```python
from build123d import *

# Parameters (mm, degrees)
SKETCH1_W           = 20
SKETCH1_H           = 50
BOSS_EXTRUDE1_DEPTH = 3
SKETCH2_W           = 50
SKETCH2_H           = 45
SKETCH2_R           = 3.5
BOSS_EXTRUDE2_DEPTH = 3


with BuildPart() as part:
    # Sketch1 → Boss-Extrude1 (new body)
    with BuildSketch(Plane(origin=(0, 0, 0), x_dir=(1, 0, 0), z_dir=(0, 1, 0))):
        Rectangle(SKETCH1_W, SKETCH1_H)
    extrude(amount=BOSS_EXTRUDE1_DEPTH)

    # Sketch2 → Boss-Extrude2 (add)
    with BuildSketch(Plane(origin=(10, 0, 0), x_dir=(0, 0, -1), z_dir=(1, 0, 0))):
        with Locations((0, 22.5)):
            Rectangle(SKETCH2_W, SKETCH2_H)
        with Locations((0, 29)):
            Circle(SKETCH2_R, mode=Mode.SUBTRACT)
    extrude(amount=BOSS_EXTRUDE2_DEPTH)


solid = part.part
```
Can you work these out from the model? Positions are in its coordinate system, mm. A direction names the side the tool comes from. Round coordinates to 2 decimals unless told otherwise and drop trailing zeros. Loops run counter-clockwise (first coordinate to the right, second up) from the corner with the lowest first, then second, coordinate; pieces in that order, holes last.
Item 1: Will these pins go through, and if not, where does the flat tip stop? pin 1 Ø1.5 at (y, z) = (34.5, 7) entering from -X; pin 2 Ø5 at (x, z) = (4, 2) entering from +Y.
Item 2: Suppose I cut it at C-C, the plane z = 15. Write out the boundary of the cut face in (x, y), then the cut area to 3 significant figures.
Item 3: Suppose I cut it at B-B, the plane z = 0. Write out the boundary of the cut face in (x, y), then the cut area to 3 significant figures.
Item 4: Which directions (+Z, -Z, +X, -X, +Y, -Y) give clear straight access to the entire face, cutting with the end or side of a thin tool? Please do faces 1 (the flat face through (10, 24, 0)), 2 (the flat face through (-10, 1, 0)).
Item 5: Please list where these lines run through material, in increasing order: L1, parallel to Y at x = 12, z = 0; L2, parallel to X at y = 19.5, z = 7.5; L3, parallel to Y at x = 7, z = 9.
Item 6: If we mould it in two halves opening along Y, with no side actions, what happens to faces 3 (the flat face through (1, 0, 0)), 4 (the flat face through (13, 23, 0)), 5 (the cylindrical face through (11.48, 32.47, 0.46))? For each: +Y half, -Y half, draft (parallel to the pull), parting line (faces both ways), or undercut.
Item 7: Suppose I cut it at A-A, the plane y = 29. Write out the boundary of the cut face in (x, z), then the cut area to 3 significant figures.
Item 8: Suppose I cut it at D-D, the plane x = -4.5. Write out the boundary of the cut face in (y, z), then the cut area to 3 significant figures.
Reported:
1. pin 1: stops at x = 10
1. pin 2: stops at y = 3
2. outline: (-10, 0) - (13, 0) - (13, 45) - (10, 45) - (10, 3) - (-10, 3) - close
2. area: 195 mm2
3. outline: (-10, 0) - (13, 0) - (13, 25.5) - (10, 25.5) - (10, 3) - (-10, 3) - close; (10, 32.5) - (13, 32.5) - (13, 45) - (10, 45) - close
3. area: 174 mm2
4. face 1: +Z, -Z, -X, +Y
4. face 2: +Z, -Z, -X, +Y, -Y
5. L1: y = 0 to 25.5, 32.5 to 45
5. L2: x = 10 to 13
5. L3: y = 0 to 3
6. face 3: -Y half
6. face 4: draft
6. face 5: undercut
7. outline: (10, -25) - (13, -25) - (13, -3.5) - (10, -3.5) - close; (10, 3.5) - (13, 3.5) - (13, 25) - (10, 25) - close
7. area: 129 mm2
8. outline: (0, -25) - (3, -25) - (3, 25) - (0, 25) - close
8. area: 150 mm2
